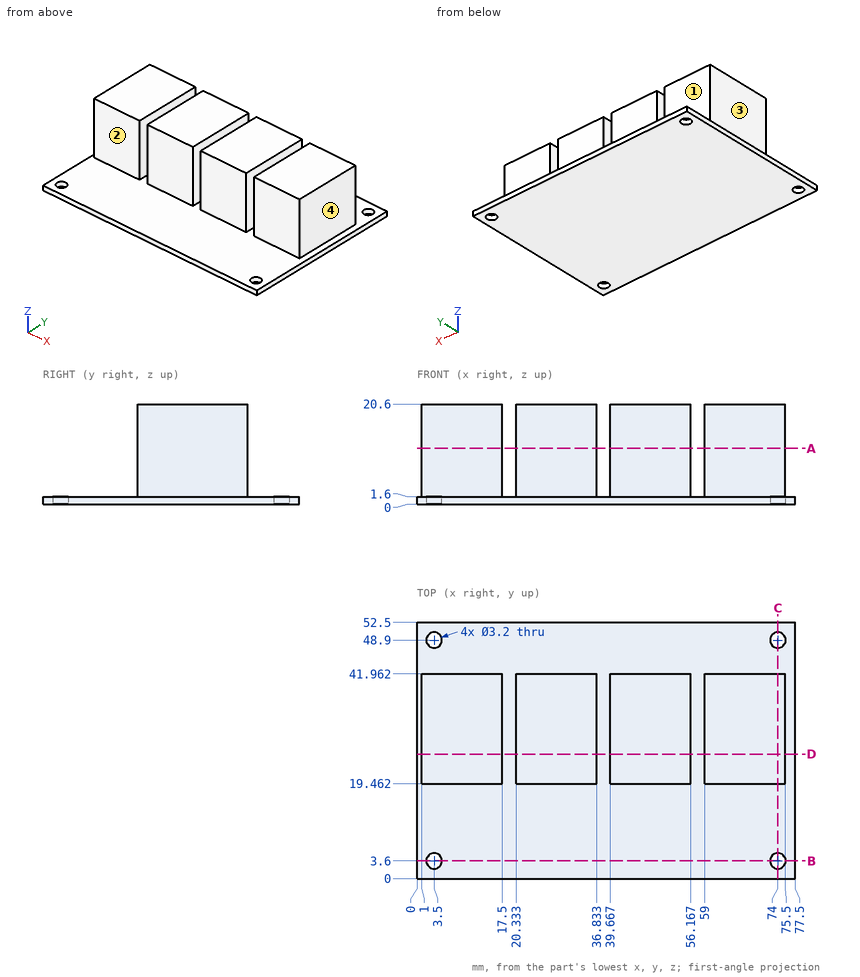
Geometry check sheet. Reference: drawing and pictorial views, mm from the part's lowest x, y, z. A direction names the side the tool comes from. Coordinates: 2 decimals unless noted, no trailing zeros. Loops run counter-clockwise (first coordinate to the right, second up) from the corner with the lowest first, then second, coordinate; pieces in that order, holes last. Notation, with made-up numbers: (-12, -23.5) - (40, -23.5) arc R30 ccw to (40, 9.5) - close; hole circle Ø6 at (-16, 39.25). An arc over 180 degrees is marked (long way). Return JSON: item names as keys, results as strings.
1. Section check A-A, the plane z = 11.5. Record the boundary of the cut face in (x, y), then the cut area to 4 significant figures.
Established:
{"outline": "(1, 19.46) - (17.5, 19.46) - (17.5, 41.96) - (1, 41.96) - close; (20.33, 19.46) - (36.83, 19.46) - (36.83, 41.96) - (20.33, 41.96) - close; (39.67, 19.46) - (56.17, 19.46) - (56.17, 41.96) - (39.67, 41.96) - close; (59, 19.46) - (75.5, 19.46) - (75.5, 41.96) - (59, 41.96) - close", "area": "1,485 mm2"}
2. Section check B-B, the plane y = 3.6. Record the boundary of the cut face in (x, z), then the cut area to 3 significant figures.
Established:
{"outline": "(0, 0) - (1.9, 0) - (1.9, 1.6) - (0, 1.6) - close; (5.1, 0) - (72.4, 0) - (72.4, 1.6) - (5.1, 1.6) - close; (75.6, 0) - (77.5, 0) - (77.5, 1.6) - (75.6, 1.6) - close", "area": "114 mm2"}
3. Section check D-D, the plane y = 25.5. Record the boundary of the cut face in (x, z), then the cut area to 3 significant figures.
Established:
{"outline": "(0, 0) - (77.5, 0) - (77.5, 1.6) - (75.5, 1.6) - (75.5, 20.6) - (59, 20.6) - (59, 1.6) - (56.17, 1.6) - (56.17, 20.6) - (39.67, 20.6) - (39.67, 1.6) - (36.83, 1.6) - (36.83, 20.6) - (20.33, 20.6) - (20.33, 1.6) - (17.5, 1.6) - (17.5, 20.6) - (1, 20.6) - (1, 1.6) - (0, 1.6) - close", "area": "1,380 mm2"}
4. Go/stop test with flat-tipped pins: pin 1 (4 mm diameter, centred on x = 62, z = 5, fed in from +Y); pin 2 (2 mm diameter, centred on y = 33.5, z = 17, fed in from -X); pin 3 (4 mm diameter, centred on x = 74, y = 48.9, fed in from -Z); pin 4 (5.5 mm diameter, centred on y = 31, z = 13.5, fed in from +X). Record where each tip stops, or that it passes through.
Established:
{"pin 1": "stops at y = 41.96", "pin 2": "stops at x = 1", "pin 3": "stops at z = 0", "pin 4": "stops at x = 75.5"}
5. Tool access check on the marked faces 1, 2, 3 and 4. Record the directions out of +Z, -Z, +X, -X, +Y, -Y that give a thin tool (end or side, any length) a straight path to the whole face; none if there is none.
Established:
{"face 1": "+Z, +X, -X, +Y", "face 2": "+Z, +X, -X, -Y", "face 3": "+Z, -X, +Y, -Y", "face 4": "+Z, +X, +Y, -Y"}
6. Section check C-C, the plane x = 74. Record the boundary of the cut face in (y, z), then the cut area to 3 significant figures.
Established:
{"outline": "(0, 0) - (2, 0) - (2, 1.6) - (0, 1.6) - close; (5.2, 0) - (47.3, 0) - (47.3, 1.6) - (41.96, 1.6) - (41.96, 20.6) - (19.46, 20.6) - (19.46, 1.6) - (5.2, 1.6) - close; (50.5, 0) - (52.5, 0) - (52.5, 1.6) - (50.5, 1.6) - close", "area": "501 mm2"}
7. Thickness scan on L1, parallel to X at y = 34.5, z = 13; L2, parallel to Y at x = 3.5, z = 0.6; L3, parallel to Z at x = 8.5, y = 48. Record the ranges inside material, lowest first.
Established:
{"L1": "x = 1 to 17.5, 20.33 to 36.83, 39.67 to 56.17, 59 to 75.5", "L2": "y = 0 to 2, 5.2 to 47.3, 50.5 to 52.5", "L3": "z = 0 to 1.6"}
